Input: part model. Units: mm. Frame: model coordinates. Face numbers are marked on the shaded views. A direction names the side the tool comes from. Round coordinates to 2 decimals unless told otherwise and drop trailing zeros. Loops run counter-clockwise (first coordinate to the right, second up) from the corner with the lowest first, then second, coordinate; pieces in that order, holes last. Notation, with made-up numbers: (62, -24) - (71, -24) arc R20 cw to (71, 11) - close; hole circle Ø6 at (49, 68.5). An arc over 180 degrees is marked (long way). One line per question, with ' | ' between items. Start each with the question number.
Item 1: Section B-B, the plane x = 0. Return loops of the section in (y, z), plus the area to 3 significant figures.
Item 2: Section A-A, the plane y = 0. Return loops of the section in (x, z), plus the area to 3 significant figures.
Item 3: First-contact query: pin 1 (2 mm diameter, centred on x = -3.5, y = 4.5, fed in from -Z); pin 2 (6 mm diameter, centred on x = 1.5, z = -7, fed in from +Y); pin 3 (3 mm diameter, centred on x = -4.5, z = -6, fed in from -Y). Flat tips, straight axial feed; report the tip coordinate or a pass-through.
Item 4: Section D-D, the plane y = 8.5. Return loops of the section in (x, z), plus the area to 3 significant figures.
Item 5: Set-up query: the marked faces 4, 5 and 6. Return all of +Z, -Z, +X, -X, +Y, -Y with unobstructed straight access to the full face (end or side cutting, diameter ignored); none if empty.
Item 6: Draft query along X for the marked faces 1, 2 and 3. Return one class per face: pulls with the +X half, pulls with the -X half, needs draft (parallel to the pull), parting line crosses it, or undercut.
Item 7: Section C-C, the plane y = 14.5. Return loops of the section in (x, z), plus the area to 3 significant figures.
Item 8: Material intervals for line 1 along Y through (x, z) = (-1, 0); line 2 along Y through (x, z) = (0, 6.5); line 3 along Y through (x, z) = (6.25, 4.75), sorted ascending.
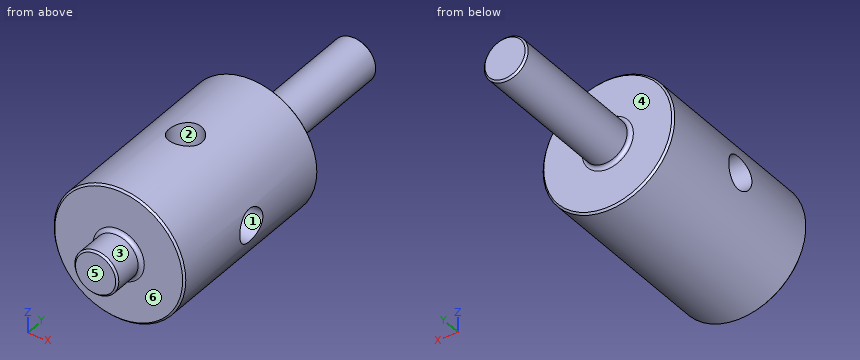
```python
from build123d import *

# Parameters (mm, degrees)
FURO_DE_DI_METRO_4_5_4_5_2_D = 4.5
ESBO_O8_W                    = 2.25
ESBO_O8_H                    = 9
FILLET1_R                    = 0.5
CHAMFER1_SIZE                = 0.25
CHAMFER4_SIZE                = 0.25


with BuildPart() as part:
    # Esboço1 → Revolução1 (revolve)
    with BuildSketch(Plane.XY):
        Polygon((0, 33), (3, 33), (3, 13), (9, 13), (9, -13), (3, -13), (3, -17.5), (0, -17.5), (0, 0), align=None)
    revolve(axis=Axis((0, 0, 0), (0, 1, 0)))

    # Furo de diâmetro Ø4.5 (4.5)2 (through all)
    with Locations(Plane(origin=(-9, 0, 0), x_dir=(0, 0, -1), z_dir=(-1, 0, 0))):
        with Locations((0, 0)):
            Hole(FURO_DE_DI_METRO_4_5_4_5_2_D / 2)

    # Esboço8 → Furo de diâmetro Ø4.5 (4.5)1 (revolve, cut)
    with BuildSketch(Plane(origin=(0, 0, 9), x_dir=(0, -1, 0), z_dir=(1, 0, 0))):
        with Locations((1.125, 4.5)):
            Rectangle(ESBO_O8_W, ESBO_O8_H)
    revolve(axis=Axis((0, 0, 15.35), (0, 0, -1)), mode=Mode.SUBTRACT)

    # Fillet1
    fillet1_edges = [part.edges().sort_by_distance(p)[0] for p in [
        (-3, -13, 0),
        (-3, 13, 0),
    ]]
    fillet(fillet1_edges, radius=FILLET1_R)

    # Chamfer1
    chamfer1_edges = [part.edges().sort_by_distance(p)[0] for p in [
        (-3, -17.5, 0),
        (-3, 33, 0),
    ]]
    chamfer(chamfer1_edges, length=CHAMFER1_SIZE)

    # Chamfer4
    chamfer4_edges = [part.edges().sort_by_distance(p)[0] for p in [
        (-9, -13, 0),
        (-9, 13, 0),
    ]]
    chamfer(chamfer4_edges, length=CHAMFER4_SIZE)


solid = part.part
```
Return value:
1) outline: (-17.5, -2.75) - (-17.25, -3) - (-13.5, -3) arc R0.5 cw to (-13, -3.5) - (-13, -8.75) - (-12.75, -9) - (12.75, -9) - (13, -8.75) - (13, -3.5) arc R0.5 cw to (13.5, -3) - (32.75, -3) - (33, -2.75) - (33, 2.75) - (32.75, 3) - (13.5, 3) arc R0.5 cw to (13, 3.5) - (13, 8.75) - (12.75, 9) - (2.25, 9) - (2.25, 0) arc R2.25 cw to (-2.25, 0) - (-2.25, 9) - (-12.75, 9) - (-13, 8.75) - (-13, 3.5) arc R0.5 cw to (-13.5, 3) - (-17.25, 3) - (-17.5, 2.75) - close | area: 567 mm2
2) outline: (-8.71, -2.25) arc R9 ccw to (8.71, -2.25) - close; (-8.71, 2.25) - (-2.25, 2.25) - (-2.25, 8.71) arc R9 ccw to start; (2.25, 2.25) - (8.71, 2.25) arc R9 ccw to (2.25, 8.71) - close | area: 144 mm2
3) pin 1: z = -8.65 | pin 2: y = 13 | pin 3: y = -13
4) outline: circle Ø18 at (0, 0) | area: 254 mm2
5) face 4: +Y | face 5: +Z, -Z, +X, -X, -Y | face 6: -Y
6) face 1: needs draft | face 2: undercut | face 3: parting line crosses it
7) outline: circle Ø6 at (0, 0) | area: 28.3 mm2
8) line 1: -17.5 to -2.25, 2.25 to 33 | line 2: -13 to -2.25, 2.25 to 13 | line 3: -13 to 13
